Geometry: final body of the model. Coordinates: model frame, mm. A direction names the side the tool comes from. Coordinates: 2 decimals unless noted, no trailing zeros. Write each loop counter-clockwise with the first axis right and the second up, starting at its lowest first coordinate (ties: lowest second). Pieces come first, ordered by that corner, then holes. Notation, with made-up numbers: (29, 40.5) -> (61, 40.5) arc R14 ccw to (61, 64.5) -> close; hole circle Ø8 at (84.25, 4.25). An arc over 180 degrees is marked (long way). One line per item, written item: value. Start each with the question number.
from build123d import *

# Parameters (mm, degrees)
F0_W      = 355.6
F0_H      = 38.1
F1_DEPTH  = 38.1
F2_W      = 38.1
F2_H      = 38.1
F3_DEPTH  = 381
F4_W      = 355.6
F4_H      = 38.1
F5_DEPTH  = 304.8
F7_DEPTH  = 38.1
F9_DEPTH  = 38.1
F10_R     = 88.9
F11_DEPTH = 38.1


with BuildPart() as f1:
    # F0 (on Front) → F1 (new body)
    with BuildSketch(Plane.XZ):
        Polygon((-47.268543, 0), (-85.368543, 0), (-85.368543, -1676.4), (-47.268543, -1676.4), (-47.268543, -800.1), (-47.268543, -762), (-47.268543, -38.1), align=None)
        with Locations((130.531457, -19.05)):
            Rectangle(F0_W, F0_H)
        Polygon((346.431457, 0), (308.331457, 0), (308.331457, -38.1), (308.331457, -762), (308.331457, -800.1), (308.331457, -1676.4), (346.431457, -1676.4), align=None)
        with Locations((130.531457, -781.05)):
            Rectangle(F0_W, F0_H)
    extrude(amount=F1_DEPTH)

    # F2 (on face) → F3 (join)
    with BuildSketch(Plane(origin=(0, 0, 0), x_dir=(-1, 0, 0), z_dir=(0, 1, 0))):
        with Locations((-327.381457, -781.05)):
            Rectangle(F2_W, F2_H)
        with Locations((66.318543, -781.05)):
            Rectangle(F2_W, F2_H)
    extrude(amount=F3_DEPTH)

    # F4 (on face) → F5 (join)
    with BuildSketch(Plane.XZ.offset(38.1)):
        Polygon((-47.268543, 0), (-85.368543, 0), (-85.368543, -800.1), (-47.268543, -800.1), (-47.268543, -38.1), align=None)
        with Locations((130.531457, -19.05)):
            Rectangle(F4_W, F4_H)
        Polygon((346.431457, 0), (308.331457, 0), (308.331457, -38.1), (308.331457, -800.1), (346.431457, -800.1), align=None)
    extrude(amount=F5_DEPTH)

    # F6 (on face) → F7 (cut)
    with BuildSketch(Plane(origin=(-85.368543, 0, 0), x_dir=(0, -1, 0), z_dir=(-1, 0, 0))):
        Polygon((342.9, 0), (38.1, -800.1), (342.9, -800.1), align=None)
    extrude(amount=-F7_DEPTH, mode=Mode.SUBTRACT)

    # F8 (on face) → F9 (cut)
    with BuildSketch(Plane.YZ.offset(346.431457)):
        Polygon((-342.9, -800.1), (-38.1, -800.1), (-342.9, 0), align=None)
    extrude(amount=-F9_DEPTH, mode=Mode.SUBTRACT)

    # F10 (on face) → F11 (cut)
    with BuildSketch(Plane.XY):
        with Locations((130.531457, -215.9)):
            Circle(F10_R)
    extrude(amount=-F11_DEPTH, mode=Mode.SUBTRACT)


solid = f1.part
Q1. First-contact query: P1, Ø11.5, axis at x = 97, z = -788, coming from the +Y side; P2, Ø11.5, axis at x = 335.5, y = 202, coming from the +Z side; P3, Ø4, axis at x = -41, y = -252, coming from the -Z side. Flat tips, straight axial feed; report the tip coordinate or a pass-through.
Q2. Draft query along Z for faces 5 (the flat face through (128, 0, -781)), 6 (the flat face through (-47.269, -125, -340)), 7 (the flat face through (-66, 188, -800.1)). Return one class per face: pulls with the +Z half, pulls with the -Z half, needs draft (parallel to the pull), parting line crosses it, or undercut.
Q3. Cut plane C-C on x = 136.5. Output: boundary loops of the cut face in (y, z).
Q4. Access query for faces 1 (the flat face through (128, -19, -800.1)), 2 (the flat face through (128, -38.1, -781)), 3 (the flat face through (327, -38.1, -1232)), 4 (the flat face through (128, -19, -762)). Directions: +Z, -Z, +X, -X, +Y, -Y. A direction counts if a zero-diameter tool reaches every point of the face in a straight line with its end or side. Return the directions, or none.
Q5. Cut plane D-D on z = -695. Output: boundary loops of the cut face in (x, y), and give its area (3 significant figures).
Q6. Line query: L1, parallel to X at y = -215, z = -30; L2, parallel to Y at x = 293.5, z = -794.5; L3, parallel to Z at x = 285, y = -32.5. Output: solid intervals per line, ascending. Write a range as from..to.
Q7. Cut plane A-A on z = -1522. Output: boundary loops of the cut face in (x, y), and give its area (3 significant figures).
Q8. Cut plane B-B on y = -215.9. Output: boundary loops of the cut face in (x, z) (3 decimals).
Solution:
1. P1: y = 0
1. P2: z = -762
1. P3: z = -38.1
2. face 5: needs draft
2. face 6: undercut
2. face 7: pulls with the -Z half
3. outline: (-342.9, -38.1) -> (-304.6, -38.1) -> (-304.6, 0) -> (-342.9, 0) -> close; (-127.2, -38.1) -> (0, -38.1) -> (0, 0) -> (-127.2, 0) -> close; (-38.1, -800.1) -> (0, -800.1) -> (0, -762) -> (-38.1, -762) -> close
4. face 1: -Z, +Y, -Y
4. face 2: -Z, -Y
4. face 3: -Z, +X, -X, -Y
4. face 4: +Y, -Y
5. outline: (-85.37, -78.14) -> (-47.27, -78.14) -> (-47.27, 0) -> (-85.37, 0) -> close; (308.33, -78.14) -> (346.43, -78.14) -> (346.43, 0) -> (308.33, 0) -> close
5. area: 5,950 mm²
6. L1: -85.37..41.64, 219.43..346.43
6. L2: -38.1..0
6. L3: -800.1..-762, -38.1..0
7. outline: (-85.37, -38.1) -> (-47.27, -38.1) -> (-47.27, 0) -> (-85.37, 0) -> close; (308.33, -38.1) -> (346.43, -38.1) -> (346.43, 0) -> (308.33, 0) -> close
7. area: 2,900 mm²
8. outline: (-85.369, -333.375) -> (-47.269, -333.375) -> (-47.269, -38.1) -> (41.631, -38.1) -> (41.631, 0) -> (-85.369, 0) -> close; (219.431, -38.1) -> (308.331, -38.1) -> (308.331, -333.375) -> (346.431, -333.375) -> (346.431, 0) -> (219.431, 0) -> close
